```python
from build123d import *

# Parameters (mm, degrees)
F1_DEPTH = 5
F2_R     = 2
F3_T     = -1.6


with BuildPart() as f1:
    # F0 (on Top) → F1 (new body)
    with BuildSketch(Plane.XY):
        Polygon((9.814955, 21.2), (-3.637307, -2.1), (20.264994, -2.1), (33.717256, 21.2), align=None)
        Polygon((19.052559, 0), (0, 0), (11.02739, 19.1), (30.079949, 19.1), align=None, mode=Mode.SUBTRACT)
        Polygon((11.02739, 19.1), (0, 0), (19.052559, 0), (30.079949, 19.1), align=None)
    extrude(amount=F1_DEPTH)

    # F2
    f2_edges = [f1.edges().sort_by_distance(p)[0] for p in [
        (-3.637307, -2.1, 2.5),
        (20.264994, -2.1, 2.5),
        (33.717256, 21.2, 2.5),
        (9.814955, 21.2, 2.5),
    ]]
    fillet(f2_edges, radius=F2_R)

    # F3
    f3_openings = [f1.faces().sort_by_distance(p)[0] for p in [
        (15.039975, 9.55, 5),
        (15.039975, 9.55, 0),
    ]]
    offset(amount=F3_T, openings=f3_openings)


solid = f1.part
```
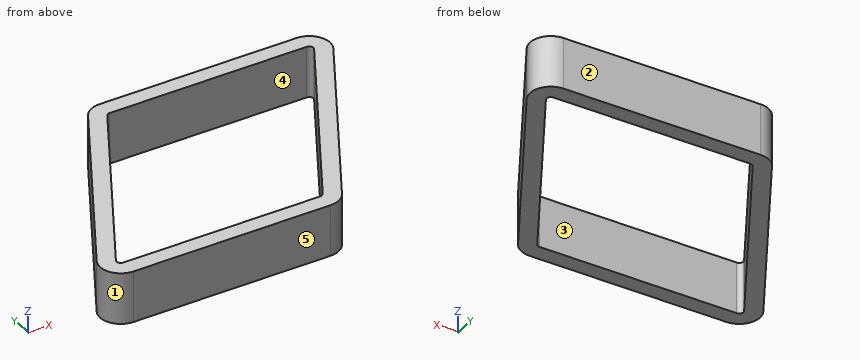
The listing builds one solid part. Answer for the finished solid, in the listing's coordinates (mm). Face numbers are marked on the shaded views. A direction names the side the tool comes from. Coordinates: 2 decimals unless noted, no trailing zeros. Write each loop counter-clockwise with the first axis right and the second up, starting at its lowest first coordinate (ties: lowest second). Pieces come first, ordered by that corner, then holes. Notation, with made-up numbers: (61, 0) - (101, 0) arc R17 ccw to (101, 31) - close; hole circle Ø2 at (30, 22). An arc over 180 degrees is marked (long way). One line per item, written item: value.
1) Find section B-B (z = 0.65). Give the vertices of the cut face in (x, y).
Geometry check:
outline: (-1.91, 0.9) arc R2 ccw to (-0.17, -2.1) - (19.11, -2.1) arc R2 ccw to (20.84, -1.1) - (31.99, 18.2) arc R2 ccw to (30.25, 21.2) - (10.97, 21.2) arc R2 ccw to (9.24, 20.2) - close; hole (-0.52, 0.1) arc R0.4 ccw to (-0.17, -0.5) - (19.11, -0.5) arc R0.4 ccw to (19.46, -0.3) - (30.6, 19) arc R0.4 ccw to (30.25, 19.6) - (10.97, 19.6) arc R0.4 ccw to (10.62, 19.4) - close
2) For a pull along X with two mould halves and no side action, classify the marked faces 1, 2 and 3 as pulls with the +X half, pulls with the -X half, needs draft (parallel to the pull), parting line crosses it, or undercut.
Geometry check:
face 1: pulls with the -X half
face 2: needs draft
face 3: undercut
3) Each of these flat-tipped pins is pushed along its axis until it touches: pin 1 Ø3 at (y, z) = (8, 1.5) entering from +X; pin 2 Ø3 at (y, z) = (15, 3) entering from +X; pin 3 Ø2 at (y, z) = (2.5, 1.5) entering from -X. Where does it stop, or does it pass through?
Geometry check:
pin 1: stops at x = 26.96
pin 2: stops at x = 31
pin 3: stops at x = -1.56
4) Consider line 1 along Y through (x, z) = (15.5, 0.8); line 2 along X through (y, z) = (1.25, 1.7); line 3 along Y through (x, z) = (3.5, 4.85). Determine where each line is inside the solid, lowest interval first. Write a range as from..to.
Geometry check:
line 1: y = -2.1..-0.5, 19.6..21.2
line 2: x = -1.7..0.14, 20.35..22.2
line 3: y = -2.1..-0.5, 7.06..10.26
5) Find section C-C (y = 4). Give the vertices of the cut face in (x, z), and give its area (3 significant figures).
Geometry check:
outline: (-0.12, 0) - (1.73, 0) - (1.73, 5) - (-0.12, 5) - close; (21.94, 0) - (23.79, 0) - (23.79, 5) - (21.94, 5) - close
area: 18.5 mm2
6) Find section A-A (x = 13.5). Give the vertices of the cut face in (y, z).
Geometry check:
outline: (-2.1, 0) - (-0.5, 0) - (-0.5, 5) - (-2.1, 5) - close; (19.6, 0) - (21.2, 0) - (21.2, 5) - (19.6, 5) - close
7) A tool of negligible diameter and unlimited length cuts with its end or side. For the marked faces 4 and 5, from which of +Z, -Z, +X, -X, +Y, -Y can it reach the whole face along a straight path? Write none if from no direction.
Geometry check:
face 4: +Z, -Z
face 5: +Z, -Z, +X, -X, -Y
